```python
from build123d import *

# Parameters (mm, degrees)
F1_DEPTH = 6.35
F2_DEPTH = 19.05
F4_DEPTH = 127
F5_SIZE  = 10.16


with BuildPart() as f1:
    # F0 (on Top) → F1 (new body)
    with BuildSketch(Plane.XY):
        with BuildLine():
            Line((50.8, 61.6115713388), (50.8, 79.375))
            Line((50.8, 79.375), (38.1, 92.075))
            Line((38.1, 92.075), (-38.1, 92.075))
            Line((-38.1, 92.075), (-50.8, 79.375))
            Line((-50.8, 79.375), (-50.8, -79.375))
            Line((-50.8, -79.375), (-38.1, -92.075))
            Line((-38.1, -92.075), (38.1, -92.075))
            Line((38.1, -92.075), (48.2682762921, -86.9839524408))
            ThreePointArc((48.2682762921, -86.9839524408), (50.5095218971, -85.1103601516), (53.3524144382, -84.4384286612))
            Line((53.3524144382, -84.4384286612), (107.95, -84.4384286612))
            ThreePointArc((107.95, -84.4384286612), (112.4401280605, -82.5785567218), (114.3, -78.0884286612))
            Line((114.3, -78.0884286612), (114.3, 48.9115713388))
            ThreePointArc((114.3, 48.9115713388), (112.4401280605, 53.4016993993), (107.95, 55.2615713388))
            Line((107.95, 55.2615713388), (57.15, 55.2615713388))
            ThreePointArc((57.15, 55.2615713388), (52.6598719395, 57.1214432782), (50.8, 61.6115713388))
        make_face()
        with BuildLine():
            ThreePointArc((-44.45, 79.375), (-42.5901280605, 83.8651280605), (-38.1, 85.725))
            Line((-38.1, 85.725), (38.1, 85.725))
            ThreePointArc((38.1, 85.725), (42.5901280605, 83.8651280605), (44.45, 79.375))
            Line((44.45, 79.375), (44.45, -79.375))
            ThreePointArc((44.45, -79.375), (42.5901280605, -83.8651280605), (38.1, -85.725))
            Line((38.1, -85.725), (-38.1, -85.725))
            ThreePointArc((-38.1, -85.725), (-42.5901280605, -83.8651280605), (-44.45, -79.375))
            Line((-44.45, -79.375), (-44.45, 79.375))
        make_face(mode=Mode.SUBTRACT)
        with BuildLine():
            Line((101.6, -78.0884286612), (57.15, -78.0884286612))
            ThreePointArc((57.15, -78.0884286612), (52.6598719395, -76.2285567218), (50.8, -71.7384286612))
            Line((50.8, -71.7384286612), (50.8, 42.5615713388))
            ThreePointArc((50.8, 42.5615713388), (52.6598719395, 47.0516993993), (57.15, 48.9115713388))
            Line((57.15, 48.9115713388), (101.6, 48.9115713388))
            ThreePointArc((101.6, 48.9115713388), (106.0901280605, 47.0516993993), (107.95, 42.5615713388))
            Line((107.95, 42.5615713388), (107.95, -71.7384286612))
            ThreePointArc((107.95, -71.7384286612), (106.0901280605, -76.2285567218), (101.6, -78.0884286612))
        make_face(mode=Mode.SUBTRACT)
        Polygon((38.1, 85.725), (-38.1, 85.725), (-44.45, 79.375), (-44.45, -79.375), (-38.1, -85.725), (38.1, -85.725), (44.45, -79.375), (44.45, 79.375), align=None)
        with BuildLine():
            ThreePointArc((50.8, -71.7384286612), (52.6598719395, -76.2285567218), (57.15, -78.0884286612))
            Line((57.15, -78.0884286612), (101.6, -78.0884286612))
            ThreePointArc((101.6, -78.0884286612), (106.0901280605, -76.2285567218), (107.95, -71.7384286612))
            Line((107.95, -71.7384286612), (107.95, 42.5615713388))
            ThreePointArc((107.95, 42.5615713388), (106.0901280605, 47.0516993993), (101.6, 48.9115713388))
            Line((101.6, 48.9115713388), (57.15, 48.9115713388))
            ThreePointArc((57.15, 48.9115713388), (52.6598719395, 47.0516993993), (50.8, 42.5615713388))
            Line((50.8, 42.5615713388), (50.8, -71.7384286612))
        make_face()
    extrude(amount=F1_DEPTH)

    # F0 (on Top) → F2 (join)
    with BuildSketch(Plane.XY):
        with BuildLine():
            Line((50.8, 61.6115713388), (50.8, 79.375))
            Line((50.8, 79.375), (38.1, 92.075))
            Line((38.1, 92.075), (-38.1, 92.075))
            Line((-38.1, 92.075), (-50.8, 79.375))
            Line((-50.8, 79.375), (-50.8, -79.375))
            Line((-50.8, -79.375), (-38.1, -92.075))
            Line((-38.1, -92.075), (38.1, -92.075))
            Line((38.1, -92.075), (48.2682762921, -86.9839524408))
            ThreePointArc((48.2682762921, -86.9839524408), (50.5095218971, -85.1103601516), (53.3524144382, -84.4384286612))
            Line((53.3524144382, -84.4384286612), (107.95, -84.4384286612))
            ThreePointArc((107.95, -84.4384286612), (112.4401280605, -82.5785567218), (114.3, -78.0884286612))
            Line((114.3, -78.0884286612), (114.3, 48.9115713388))
            ThreePointArc((114.3, 48.9115713388), (112.4401280605, 53.4016993993), (107.95, 55.2615713388))
            Line((107.95, 55.2615713388), (57.15, 55.2615713388))
            ThreePointArc((57.15, 55.2615713388), (52.6598719395, 57.1214432782), (50.8, 61.6115713388))
        make_face()
        with BuildLine():
            ThreePointArc((-44.45, 79.375), (-42.5901280605, 83.8651280605), (-38.1, 85.725))
            Line((-38.1, 85.725), (38.1, 85.725))
            ThreePointArc((38.1, 85.725), (42.5901280605, 83.8651280605), (44.45, 79.375))
            Line((44.45, 79.375), (44.45, -79.375))
            ThreePointArc((44.45, -79.375), (42.5901280605, -83.8651280605), (38.1, -85.725))
            Line((38.1, -85.725), (-38.1, -85.725))
            ThreePointArc((-38.1, -85.725), (-42.5901280605, -83.8651280605), (-44.45, -79.375))
            Line((-44.45, -79.375), (-44.45, 79.375))
        make_face(mode=Mode.SUBTRACT)
        with BuildLine():
            Line((101.6, -78.0884286612), (57.15, -78.0884286612))
            ThreePointArc((57.15, -78.0884286612), (52.6598719395, -76.2285567218), (50.8, -71.7384286612))
            Line((50.8, -71.7384286612), (50.8, 42.5615713388))
            ThreePointArc((50.8, 42.5615713388), (52.6598719395, 47.0516993993), (57.15, 48.9115713388))
            Line((57.15, 48.9115713388), (101.6, 48.9115713388))
            ThreePointArc((101.6, 48.9115713388), (106.0901280605, 47.0516993993), (107.95, 42.5615713388))
            Line((107.95, 42.5615713388), (107.95, -71.7384286612))
            ThreePointArc((107.95, -71.7384286612), (106.0901280605, -76.2285567218), (101.6, -78.0884286612))
        make_face(mode=Mode.SUBTRACT)
    extrude(amount=F2_DEPTH)

    # F3 (on Right) → F4 (cut, symmetric)
    with BuildSketch(Plane.YZ):
        with BuildLine():
            ThreePointArc((-41.7938075632, 6.35), (-29.0938075632, 4.3464379948), (-16.3938075632, 6.35))
            Line((-16.3938075632, 6.35), (-16.3938075632, 53.7061375175))
            Line((-16.3938075632, 53.7061375175), (-41.7938075632, 53.7061375175))
            Line((-41.7938075632, 53.7061375175), (-41.7938075632, 6.35))
        make_face()
    extrude(amount=F4_DEPTH, both=True, mode=Mode.SUBTRACT)

    # F5
    f5_edges = [f1.edges().sort_by_distance(p)[0] for p in [
        (111.125, -16.393808, 19.05),
        (47.625, -16.393808, 19.05),
        (-47.625, -16.393808, 19.05),
        (-47.625, -41.793808, 19.05),
        (47.625, -41.793808, 19.05),
        (111.125, -41.793808, 19.05),
    ]]
    chamfer(f5_edges, length=F5_SIZE)


solid = f1.part
```
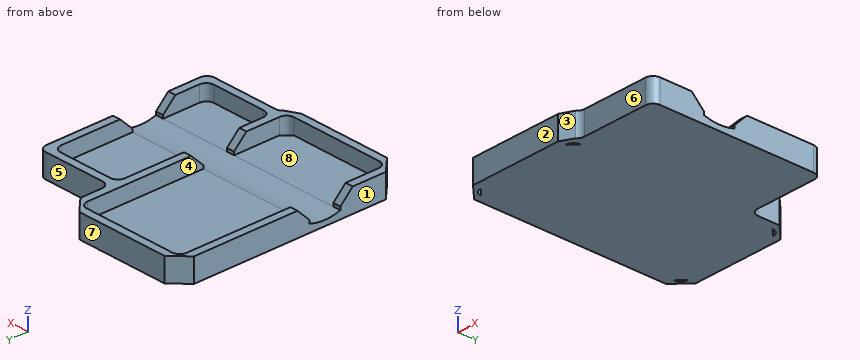
Could you check a few things on this model? Use its own coordinates, in mm. Face numbers are marked on the shaded views. A direction names the side the tool comes from. Round coordinates to 2 decimals unless told otherwise and drop trailing zeros. Order: outer loops, then holes, each group sorted by start corner. A loop starts at its lowest first (then second) coordinate and runs counter-clockwise, first axis right, second up. Notation, with made-up numbers: M 64,71.25 L 92,71.25 A33 cw 92,107.25 Z; hole C -5,54.5 d2. An arc over 180 degrees is marked long. One line per question, with ' | ' between items. Start each with the question number.
(1) Suppose I cut it at B-B on y = 72. List the corners of the cut face in (x, z) for me, then the cut area to 3 significant figures.
(2) Suppose I cut it at D-D on y = 22. List the corners of the cut face in (x, z) for me, then the cut area to 3 significant figures.
(3) For the marked faces 5, 6, 7 and 8, which set-ups out of +Z, -Z, +X, -X, +Y, -Y let a thin tool reach every point of the face, with its end or its side?
(4) Suppose I cut it at A-A on x = 76. List the corners of the cut face in (y, z) for me.
(5) Please list where these lines run through material, in increasing order: line 1 along X through (y, z) = (2, 15); line 2 along X through (y, z) = (67, 7.75).
(6) Suppose I cut it at C-C on x = 5. List the corners of the cut face in (y, z) for me (3 decimals).
(7) For P1, Ø9.5, axis at x = 80, z = 10, coming from the +Y side; P2, Ø12, axis at x = -15.5, y = -46, coming from the -Z side; P3, Ø4, axis at x = 85, z = 11.5, coming from the -Y side; P4, Ø6, axis at x = -10.5, y = -56, coming from the +Z side, each with a flat end and sliding along its axis, tell me the tip position at first contact or that it passes through.
(8) Thinking about a two-plate mould opening in X: for the marked faces 1, 2, 3 and 4, which applies, +X half, -X half, draft (parallel to the pull), parting line (faces both ways), or undercut?
Geometry results:
1) outline: M -50.8,0 L 50.8,0 L 50.8,19.05 L 44.45,19.05 L 44.45,6.35 L -44.45,6.35 L -44.45,19.05 L -50.8,19.05 Z | area: 806 mm²
2) outline: M -50.8,0 L 114.3,0 L 114.3,19.05 L 107.95,19.05 L 107.95,6.35 L 50.8,6.35 L 50.8,19.05 L 44.45,19.05 L 44.45,6.35 L -44.45,6.35 L -44.45,19.05 L -50.8,19.05 Z | area: 1,290 mm²
3) face 5: +Z, -Z, +X, +Y | face 6: +Z, -Z, +X, -Y | face 7: +Z, -Z, +X, -X, +Y | face 8: +Z
4) outline: M -84.44,0 L 55.26,0 L 55.26,19.05 L 48.91,19.05 L 48.91,6.35 L -16.39,6.35 A41.25 cw -41.79,6.35 L -78.09,6.35 L -78.09,19.05 L -84.44,19.05 Z
5) line 1: -50.8 to -44.45, 44.45 to 50.8, 107.95 to 114.3 | line 2: -50.8 to -44.45, 44.45 to 50.8
6) outline: M -92.075,0 L 92.075,0 L 92.075,19.05 L 85.725,19.05 L 85.725,6.35 L -16.394,6.35 A41.253 cw -41.794,6.35 L -85.725,6.35 L -85.725,19.05 L -92.075,19.05 Z
7) P1: y = 55.26 | P2: z = 0 | P3: y = -84.44 | P4: z = 6.35
8) face 1: -X half | face 2: draft | face 3: +X half | face 4: undercut
